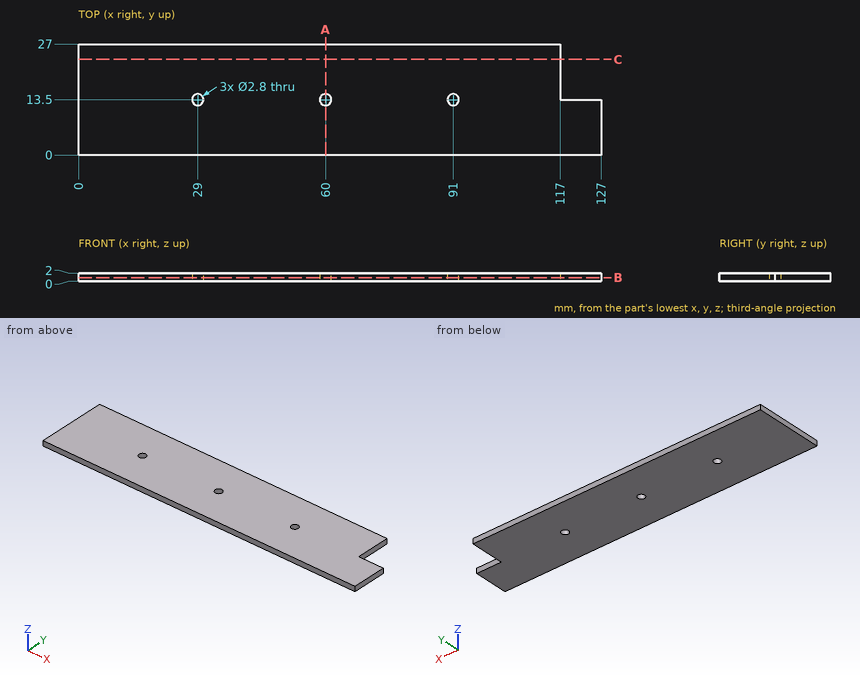
Source: three-view drawing plus pictorial views. Frame: mm from the lowest corner of the part. Give positions to 0.01 mm unless a question says otherwise; leave off trailing zeros. Order: outer loops, then holes, each group sorted by start corner. A loop starts at its lowest first (then second) coordinate and runs counter-clockwise, first axis right, second up. Notation, with made-up numbers: (-40, -21.75) - (-27, -21.75) arc R27 ccw to (-27, 6.25) - close; hole circle Ø8 at (-5.5, 56). An arc over 180 degrees is marked (long way). Answer as a JSON object with one key per item and string values. Group by question number.
Q1. Line query: probe 1 along Y at (x, z) = (29, 1.05); probe 2 along X at (y, z) = (14.25, 1.3); probe 3 along X at (y, z) = (19, 1.8). Output: solid intervals per line, ascending.
Q2. First-contact query: pin 1 Ø2.5 at (x, y) = (60, 13.5) entering from -Z; pin 2 Ø1 at (y, z) = (15, 0.5) entering from +X. Flat tips, straight axial feed; report the tip coordinate or a pass-through.
Q3. Cut plane B-B, the plane z = 0.9. Output: boundary loops of the cut face in (x, y).
Q4. Cut plane A-A, the plane x = 60. Output: boundary loops of the cut face in (y, z), then the cut area to 3 significant figures.
Q5. Cut plane C-C, the plane y = 23.25. Output: boundary loops of the cut face in (x, z), then the cut area to 3 significant figures.
Results:
{
 "1": {"probe 1": "0 to 12.1, 14.9 to 27", "probe 2": "0 to 27.82, 30.18 to 58.82, 61.18 to 89.82, 92.18 to 117", "probe 3": "0 to 117"},
 "2": {"pin 1": "through", "pin 2": "x = 117"},
 "3": {"outline": "(0, 0) - (127, 0) - (127, 13.5) - (117, 13.5) - (117, 27) - (0, 27) - close; hole circle Ø2.8 at (29, 13.5); hole circle Ø2.8 at (60, 13.5); hole circle Ø2.8 at (91, 13.5)"},
 "4": {"outline": "(0, 0) - (12.1, 0) - (12.1, 2) - (0, 2) - close; (14.9, 0) - (27, 0) - (27, 2) - (14.9, 2) - close", "area": "48.4 mm^2"},
 "5": {"outline": "(0, 0) - (117, 0) - (117, 2) - (0, 2) - close", "area": "234 mm^2"}
}
